```python
from build123d import *

# Parameters (mm, degrees)
SKETCH_1_R               = 6
SKETCH_1_R_2             = 4
EXTRUDE_1_DEPTH          = 30
EXTRUDE_2_DEPTH          = 3
EXTRUDE_2_DEPTH_BACK     = 5
SKETCH_2_R               = 9
CUT_EXTRUDE_1_DEPTH      = 33.588341474
CUT_EXTRUDE_1_DEPTH_BACK = 33.588341474
SKETCH_3_R               = 1.6
CUT_EXTRUDE_2_DEPTH      = 33.588341529
CUT_EXTRUDE_2_DEPTH_BACK = 33.588341529
SKETCH_4_R               = 1.6
FILLET_1_R               = 1


with BuildPart() as part:
    # 草图1 → 凸台-拉伸1 (new body)
    with BuildSketch(Plane(origin=(0, 0, 0), x_dir=(1, 0, 0), z_dir=(0, 1, 0))):
        with Locations(Location((0, 0, 0), (0, 0, 270))):
            Circle(SKETCH_1_R)
        with Locations(Location((0, 0, 0), (0, 0, 270))):
            Circle(SKETCH_1_R_2, mode=Mode.SUBTRACT)
    extrude(amount=EXTRUDE_1_DEPTH)

    # 草图2 → 凸台-拉伸2 (add, two sides: drawn at the far end of the back side and taken through both)
    with BuildSketch(Plane.XZ.offset(-EXTRUDE_2_DEPTH_BACK)):
        with Locations(Location((0, 0, 0), (0, 0, 270))):
            Circle(SKETCH_2_R)
    extrude(amount=EXTRUDE_2_DEPTH + EXTRUDE_2_DEPTH_BACK)

    # 草图3 → 切除-拉伸1 (cut, two sides: drawn at the far end of the back side and taken through both)
    with BuildSketch(Plane(origin=(0, 0, 0), x_dir=(0, 0, -1), z_dir=(1, 0, 0)).offset(-CUT_EXTRUDE_1_DEPTH_BACK)):
        with Locations((-6, 1)):
            Circle(SKETCH_3_R)
        with Locations((6, 1)):
            Circle(SKETCH_3_R)
    extrude(amount=CUT_EXTRUDE_1_DEPTH + CUT_EXTRUDE_1_DEPTH_BACK, mode=Mode.SUBTRACT)

    # 草图4 → 切除-拉伸2 (cut, two sides: drawn at the far end of the back side and taken through both)
    with BuildSketch(Plane.XY.offset(-CUT_EXTRUDE_2_DEPTH_BACK)):
        with Locations(Location((-6, 1, 0), (0, 0, 270))):
            Circle(SKETCH_4_R)
        with Locations(Location((6, 1, 0), (0, 0, 270))):
            Circle(SKETCH_4_R)
    extrude(amount=CUT_EXTRUDE_2_DEPTH + CUT_EXTRUDE_2_DEPTH_BACK, mode=Mode.SUBTRACT)

    # 圆角1
    fillet_1_edges = [part.edges().sort_by_distance(p)[0] for p in [
        (0, 5, -6),
        (0, 5, 9),
        (0, -3, 9),
        (0, 30, -6),
    ]]
    fillet(fillet_1_edges, radius=FILLET_1_R)


solid = part.part
```
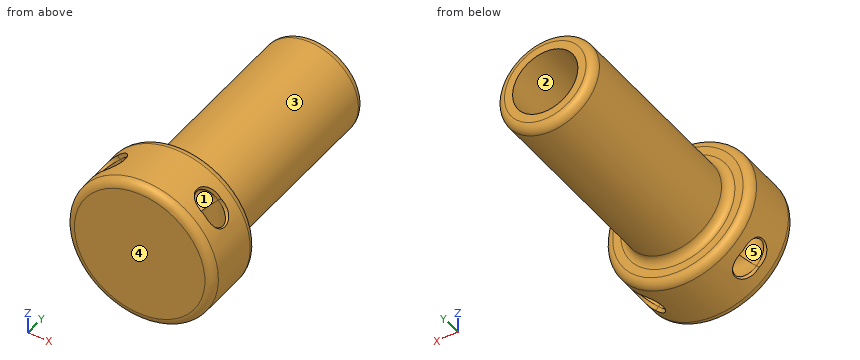
CAD build for the part. Positions are in the model's coordinates, mm. Face numbers are marked on the shaded views. A direction names the side the tool comes from. Coordinates: 2 decimals unless noted, no trailing zeros. Order: outer loops, then holes, each group sorted by start corner. A loop starts at its lowest first (then second) coordinate and runs counter-clockwise, first axis right, second up.
(1) Saw through at C-C, the plane x = 0. Write the cut outline in (y, z), and give its area (3 significant figures).
Solution:
outline: (-3, -8) arc R1 ccw to (-2, -9) - (4, -9) arc R1 ccw to (5, -8) - (5, -7) arc R1 cw to (6, -6) - (29, -6) arc R1 ccw to (30, -5) - (30, -4) - (5, -4) - (5, 4) - (30, 4) - (30, 5) arc R1 ccw to (29, 6) - (6, 6) arc R1 cw to (5, 7) - (5, 8) arc R1 ccw to (4, 9) - (-2, 9) arc R1 ccw to (-3, 8) - close; hole circle Ø3.2 at (1, -6); hole circle Ø3.2 at (1, 6)
area: 227 mm2
(2) Pin check, flat tips, straight feed: pin 1 Ø6 at (x, y) = (-6, 22) entering from -Z; pin 2 Ø3.5 at (x, y) = (-6, 1) entering from +Z; pin 3 Ø5 at (y, z) = (1, -6) entering from -X; pin 4 Ø9 at (x, z) = (0.5, 2) entering from +Y. Stop position of each tip, or through.
Solution:
pin 1: stops at z = -5.2
pin 2: stops at z = 7.93
pin 3: stops at x = -8.29
pin 4: stops at y = 30
(3) Drill centre lines: L1, parallel to Z at x = -0.25, y = 1; L2, parallel to X at y = 1, z = 3.25; L3, parallel to Z at x = 0, y = 12. Where is each one in solid material? Low to high.
Solution:
L1: z = -9 to -7.6, -4.4 to 4.4, 7.6 to 9
L2: x = -8.39 to -7.6, -4.4 to 4.4, 7.6 to 8.39
L3: z = -6 to -4, 4 to 6
(4) Which spindle directions (+Z, -Z, +X, -X, +Y, -Y) get a long thin tool onto all of the face, cutting with end or side? Do the marked faces 1 and 2. Say none if no direction does.
Solution:
face 1: +X, -X
face 2: +Y
(5) Saw through at A-A, the plane z = 0. Write the cut outline in (x, y).
Solution:
outline: (-9, -2) arc R1 ccw to (-8, -3) - (8, -3) arc R1 ccw to (9, -2) - (9, 4) arc R1 ccw to (8, 5) - (7, 5) arc R1 cw to (6, 6) - (6, 29) arc R1 ccw to (5, 30) - (4, 30) - (4, 5) - (-4, 5) - (-4, 30) - (-5, 30) arc R1 ccw to (-6, 29) - (-6, 6) arc R1 cw to (-7, 5) - (-8, 5) arc R1 ccw to (-9, 4) - close; hole circle Ø3.2 at (-6, 1); hole circle Ø3.2 at (6, 1)
(6) Saw through at D-D, the plane y = 21. Write the cut outline in (x, z), and give its area (3 significant figures).
Solution:
outline: circle Ø12 at (0, 0); hole circle Ø8 at (0, 0)
area: 62.8 mm2
(7) Saw through at B-B, the plane y = 1. Write the cut outline in (x, z), and give its area (3 significant figures).
Solution:
outline: (-7.85, -4.4) - (-7.6, -4.4) - (-7.6, 4.4) - (-7.85, 4.4) arc R9 ccw to start; (-4.4, -7.85) arc R9 ccw to (4.4, -7.85) - (4.4, -7.6) - (-4.4, -7.6) - close; (-4.4, -4.4) - (4.4, -4.4) - (4.4, 4.4) - (-4.4, 4.4) - close; (-4.4, 7.6) - (4.4, 7.6) - (4.4, 7.85) arc R9 ccw to (-4.4, 7.85) - close; (7.6, -4.4) - (7.85, -4.4) arc R9 ccw to (7.85, 4.4) - (7.6, 4.4) - close
area: 114 mm2
(8) Mould opens along Y. For the marked faces 3, 4 and 5 say: released by +Y, released by -Y, zero draft, split by the parting line, or undercut.
Solution:
face 3: zero draft
face 4: released by -Y
face 5: undercut
